```python
from build123d import *

# Parameters (mm, degrees)
F0_W       = 152.4421870708
F0_H       = 6.5507292747
F3_DEPTH   = 17.78
F4_D       = 6.35
F4_ON_F2_D = 6.35
F6_W       = 5.683042109
F6_H       = 6.1811245978
F7_DEPTH   = 25.4
F5_W       = 6.5025947988
F5_H       = 6.5507292747
F8_DEPTH   = 25.4
F10_D      = 3.81
F10_DEPTH  = 12.7
F10_TIP    = 1.1446394792
F12_D      = 3.81


with BuildPart() as f3:
    # F0 (on Front) → F3 (new body)
    with BuildSketch(Plane.XZ):
        with Locations((9.5233023167, 47.2025945783)):
            Rectangle(F0_W, F0_H)
    extrude(amount=F3_DEPTH)

    # F4 (through all)
    with Locations(Plane(origin=(0, 0, 0), x_dir=(1, 0, 0), z_dir=(0, 1, 0))):
        with Locations((-62.0040521026, -47.4707409739)):
            Hole(F4_D / 2)

    # F4 on F2 (through all)
    with Locations(Plane(origin=(0, 0, 0), x_dir=(1, 0, 0), z_dir=(0, 1, 0))):
        with Locations((80.0990313292, -47.4590882659)):
            Hole(F4_ON_F2_D / 2)

    # F6 (on face) → F7 (join)
    with BuildSketch(Plane.XZ.offset(17.78)):
        with Locations((66.0152845085, 47.3873969167)):
            Rectangle(F6_W, F6_H)
    extrude(amount=F7_DEPTH)

    # F5 (on face) → F8 (join)
    with BuildSketch(Plane.XZ.offset(17.78)):
        with Locations((-49.1894576699, 47.2025945783)):
            Rectangle(F5_W, F5_H)
    extrude(amount=F8_DEPTH)

    # F10
    with Locations(Plane(origin=(-52.4407550693, 0, 0), x_dir=(0, -1, 0), z_dir=(-1, 0, 0))):
        with Locations((38.4867973626, 47.3310947418)):
            Hole(F10_D / 2, depth=F10_DEPTH)
            with Locations((0, 0, -(F10_DEPTH + F10_TIP / 2))):  # 118° drill point
                Cone(0, F10_D / 2, F10_TIP, mode=Mode.SUBTRACT)

    # F12 (through all)
    with Locations(Plane.YZ.offset(68.856805563)):
        with Locations((-39.1976609826, 47.6043485105)):
            Hole(F12_D / 2)


solid = f3.part
```
The model under review builds one solid part; all positions refer to its coordinate system, in mm. A direction names the side the tool comes from. Coordinates: 2 decimals unless noted, no trailing zeros. Write each loop counter-clockwise with the first axis right and the second up, starting at its lowest first coordinate (ties: lowest second). Pieces come first, ordered by that corner, then holes. Notation, with made-up numbers: (39, 38) - (59, 38) arc R30 ccw to (59, 65) - close; hole circle Ø9 at (-15, 49). An arc over 180 degrees is marked (long way). Answer in a Markdown table with one row per item. Add a question column.
Q1. For faces 4 (the face through (63.174, -30, 47)), 5 (the face through (-52.441, -30, 47)), 6 (the face through (68.857, -30, 47)), list the 3-axis set-ups (+Z, -Z, +X, -X, +Y, -Y) from which the entire face can be reached by the end or side of a thin tool; tool diameter is ignored.
Q2. To check wall thickness, follow line 1 along X through (y, z) = (-6.5, 47.5); line 2 along X through (y, z) = (-22, 44.75); line 3 along X through (y, z) = (-6.5, 45.75). State the ranges of each line that lie inside material, in increasing order. Write a range as from..to.
Q3. Draft analysis for pull direction Z (two halves, no side actions). For faces 1 (the face through (79.973, -9.014, 44.287)), 2 (the face through (66, -30, 44.297)), 3 (the face through (-45.938, -30, 47)), state which applies: +Z half, -Z half, draft (parallel to the pull), parting line (faces both ways), or undercut.
Q4. Clearance check with flat-ended pins moving along their axes: pin 1 (1.9 mm diameter, centred on y = -31, z = 48, fed in from -X); pin 2 (1 mm diameter, centred on x = 69.5, z = 47, fed in from -Y); pin 3 (8 mm diameter, centred on x = -40, y = -31.5, fed in from -Z); pin 4 (2 mm diameter, centred on y = -25.5, z = 46.5, fed in from +X). State where each tip first meets the part, or that it passes through.
Q5. Consider section B-B on y = -31. Give the boundary of the cut face in (x, z), then the cut area to 3 significant figures.
Q6. Consider section C-C on x = 50. Give the boundary of the cut face in (y, z), then the cut area to 3 significant figures.
Q7. Consider section A-A on y = -12. Give the boundary of the cut face in (x, z) (3 decimals).
Answers below:
| question | item | result |
|---|---|---|
| 1 | face 4 | +Z, -Z, -Y |
| 1 | face 5 | +Z, -Z, -X, -Y |
| 1 | face 6 | +Z, -Z, +X, -Y |
| 2 | line 1 | -66.7..-65.18, -58.83..76.92, 83.27..85.74 |
| 2 | line 2 | -52.44..-45.94, 63.17..68.86 |
| 2 | line 3 | -66.7..-64.67, -59.34..77.42, 82.77..85.74 |
| 3 | face 1 | undercut |
| 3 | face 2 | -Z half |
| 3 | face 3 | draft |
| 4 | pin 1 | x = -52.44 |
| 4 | pin 2 | y = -17.78 |
| 4 | pin 3 | through |
| 4 | pin 4 | x = 68.86 |
| 5 | outline | (-52.44, 43.93) - (-45.94, 43.93) - (-45.94, 50.48) - (-52.44, 50.48) - close; (63.17, 44.3) - (68.86, 44.3) - (68.86, 50.48) - (63.17, 50.48) - close |
| 5 | area | 77.7 mm² |
| 6 | outline | (-17.78, 43.93) - (0, 43.93) - (0, 50.48) - (-17.78, 50.48) - close |
| 6 | area | 116 mm² |
| 7 | outline | (-66.698, 43.927) - (85.744, 43.927) - (85.744, 50.478) - (81.082, 50.478) arc R3.175 cw (long way) to (79.116, 50.478) - (-60.986, 50.478) arc R3.175 cw (long way) to (-63.023, 50.478) - (-66.698, 50.478) - close |
